Can you work these out from the model? Positions are in its coordinate system, mm. Coordinates: 2 decimals unless noted, no trailing zeros. Order: outer loops, then holes, each group sorted by start corner. A loop starts at its lowest first (then second) coordinate and runs counter-clockwise, first axis right, second up.
```python
from build123d import *

# Parameters (mm, degrees)
BOSS_EXTRU_1_DEPTH = 580


with BuildPart() as part:
    # Esquisse1 → Boss.-Extru.1 (new body)
    with BuildSketch(Plane(origin=(0, 0, 0), x_dir=(1, 0, 0), z_dir=(0, 1, 0))):
        Polygon((-3.535533906, 0), (-6.035533906, 2.5), (-6.035533906, 0), align=None)
        Polygon((0, 3.535533906), (-2.5, 6.035533906), (-2.5, 2.5), (-6.035533906, 2.5), (-3.535533906, 0), (0, 0), align=None)
        Polygon((0, 6.035533906), (-2.5, 6.035533906), (0, 3.535533906), align=None)
        Polygon((-2.5, 2.5), (-2.5, 6.035533906), (-6.464466094, 10), (-10, 6.464466094), (-6.035533906, 2.5), align=None)
        Polygon((-13.964466094, 0), (-13.964466094, 2.5), (-16.464466094, 0), align=None)
        Polygon((-17.5, 2.5), (-17.5, 6.035533906), (-20, 3.535533906), (-20, 0), (-16.464466094, 0), (-13.964466094, 2.5), align=None)
        Polygon((-20, 3.535533906), (-17.5, 6.035533906), (-20, 6.035533906), align=None)
        Polygon((-10, 6.464466094), (-13.535533906, 10), (-17.5, 6.035533906), (-17.5, 2.5), (-13.964466094, 2.5), align=None)
        Polygon((-6.464466094, 10), (-10, 13.535533906), (-13.535533906, 10), (-10, 6.464466094), align=None)
        Polygon((-2.5, 13.964466094), (-2.5, 17.5), (-6.035533906, 17.5), (-10, 13.535533906), (-6.464466094, 10), align=None)
        Polygon((-6.035533906, 17.5), (-2.5, 17.5), (-2.5, 13.964466094), (0, 16.464466094), (0, 20), (-3.535533906, 20), align=None)
        Polygon((0, 16.464466094), (-2.5, 13.964466094), (0, 13.964466094), align=None)
        Polygon((-6.035533906, 20), (-6.035533906, 17.5), (-3.535533906, 20), align=None)
        Polygon((-16.464466094, 20), (-13.964466094, 17.5), (-13.964466094, 20), align=None)
        Polygon((-17.5, 17.5), (-13.964466094, 17.5), (-16.464466094, 20), (-20, 20), (-20, 16.464466094), (-17.5, 13.964466094), align=None)
        Polygon((-20, 13.964466094), (-17.5, 13.964466094), (-20, 16.464466094), align=None)
        Polygon((-10, 13.535533906), (-13.964466094, 17.5), (-17.5, 17.5), (-17.5, 13.964466094), (-13.535533906, 10), align=None)
    extrude(amount=BOSS_EXTRU_1_DEPTH)


solid = part.part
```
1. Please list where these lines run through material, in increasing order: probe 1 along X at (y, z) = (422, -18); probe 2 along Z at (x, y) = (-3, 37).
Completed:
probe 1: x = -20 to -13.96, -6.04 to 0
probe 2: z = -20 to -13.46, -6.54 to 0
2. I'm going to push a flat-ended pin straight in: pin 1 (1 mm diameter, centred on y = 496, z = -13, fed in from -X). Where does the tip first touch, or does it pass through?
Completed:
pin 1: stops at x = -17.04
3. Imagine slicing it at A-A on y = 71.5. Please give me the cut outline in (x, z), then the cut area to 3 significant figures.
Completed:
outline: (-20, -20) - (-13.96, -20) - (-13.96, -17.5) - (-10, -13.54) - (-6.04, -17.5) - (-6.04, -20) - (0, -20) - (0, -13.96) - (-2.5, -13.96) - (-6.46, -10) - (-2.5, -6.04) - (0, -6.04) - (0, 0) - (-6.04, 0) - (-6.04, -2.5) - (-10, -6.46) - (-13.96, -2.5) - (-13.96, 0) - (-20, 0) - (-20, -6.04) - (-17.5, -6.04) - (-13.54, -10) - (-17.5, -13.96) - (-20, -13.96) - close
area: 258 mm2
